Read the model definition and answer for the solid it produces. Units are mm, in the model's axes. A direction names the side the tool comes from. Coordinates: 2 decimals unless noted, no trailing zeros. Write each loop counter-clockwise with the first axis right and the second up, starting at its lowest first coordinate (ties: lowest second). Pieces come first, ordered by that corner, then holes. Notation, with made-up numbers: (-13.5, 42.25) -> (4.5, 42.25) arc R21 cw to (4.5, 77.25) -> close; hole circle Ø1 at (33.25, 58.5). An arc over 180 degrees is marked (long way). Return JSON: item names as keys, results as strings.
from build123d import *

# Parameters (mm, degrees)
ESQUISSE1_R             = 4
BOSS_EXTRU_1_DEPTH      = 3
ESQUISSE2_W             = 4.5
ESQUISSE2_H             = 4.5
BOSS_EXTRU_2_DEPTH      = 9
ESQUISSE3_W             = 2.4
ESQUISSE3_H             = 2.4
ENL_V_MAT_EXTRU_1_DEPTH = 3
CONG_1_R                = 1
CONG_2_R                = 0.5


with BuildPart() as part:
    # Esquisse1 → Boss.-Extru.1 (new body)
    with BuildSketch(Plane.XY):
        Circle(ESQUISSE1_R)
    extrude(amount=BOSS_EXTRU_1_DEPTH)

    # Esquisse2 → Boss.-Extru.2 (add)
    with BuildSketch(Plane.XY.offset(3)):
        Rectangle(ESQUISSE2_W, ESQUISSE2_H)
    extrude(amount=BOSS_EXTRU_2_DEPTH)

    # Esquisse3 → Enlèv. mat.-Extru.1 (cut)
    with BuildSketch(Plane.XY.offset(12)):
        Rectangle(ESQUISSE3_W, ESQUISSE3_H)
    extrude(amount=-ENL_V_MAT_EXTRU_1_DEPTH, mode=Mode.SUBTRACT)

    # Congé1
    cong_1_edges = [part.edges().sort_by_distance(p)[0] for p in [
        (-2.25, 2.25, 7.5),
        (-2.25, -2.25, 7.5),
        (2.25, -2.25, 7.5),
        (2.25, 2.25, 7.5),
    ]]
    fillet(cong_1_edges, radius=CONG_1_R)

    # Congé2
    cong_2_edges = [part.edges().sort_by_distance(p)[0] for p in [
        (-4, 0, 0),
    ]]
    fillet(cong_2_edges, radius=CONG_2_R)


solid = part.part
1. Flat-ended cylindrical pins translate along their axes: pin 1 Ø4 at (x, z) = (2, 4.5) entering from -Y; pin 2 Ø0.8 at (x, z) = (0.5, 6) entering from -Y; pin 3 Ø3 at (x, z) = (-0.5, 5.5) entering from +Y. Find the tip coordinate at first contact, or state that the pin passes through.
Taken from the geometry:
{"pin 1": "stops at y = -3.94", "pin 2": "stops at y = -2.25", "pin 3": "stops at y = 2.25"}
2. Consider L1, parallel to Y at x = -0.25, z = 5.75; L2, parallel to Z at x = -1.5, y = -2.25. Determine where each line is inside the solid, lowest interval first.
Taken from the geometry:
{"L1": "y = -2.25 to 2.25", "L2": "z = 0 to 3"}
3. A tool of negligible diameter and unlimited length cuts with its end or side. For faces 1 (the face through (-1.949, 1.965, 7.563)), 2 (the face through (0, -2.25, 7)), 3 (the face through (0, 2.25, 7)), 4 (the face through (2.25, 0, 7)), 5 (the face through (0, -1.2, 11)), from which of +Z, -Z, +X, -X, +Y, -Y can it reach the whole face along a straight path? Write none if from no direction.
Taken from the geometry:
{"face 1": "+Z, -X, +Y", "face 2": "+Z, +X, -X, -Y", "face 3": "+Z, +X, -X, +Y", "face 4": "+Z, +X, +Y, -Y", "face 5": "+Z"}
4. For a pull along X with two mould halves and no side action, classify faces 6 (the face through (1.949, -1.965, 7.563)), 7 (the face through (-1.949, -1.965, 7.563)), 8 (the face through (1.2, 0, 11)), 9 (the face through (3, 0, 3)) as +X half, -X half, draft (parallel to the pull), parting line (faces both ways), or undercut.
Taken from the geometry:
{"face 6": "+X half", "face 7": "-X half", "face 8": "undercut", "face 9": "draft"}
5. The part is cut by section D-D (z = 8.5). Determine the outline of the cut face in (x, y), then the cut area to 3 significant figures.
Taken from the geometry:
{"outline": "(-2.25, -1.25) arc R1 ccw to (-1.25, -2.25) -> (1.25, -2.25) arc R1 ccw to (2.25, -1.25) -> (2.25, 1.25) arc R1 ccw to (1.25, 2.25) -> (-1.25, 2.25) arc R1 ccw to (-2.25, 1.25) -> close", "area": "19.4 mm2"}
6. The part is cut by section A-A (z = 11.25). Determine the outline of the cut face in (x, y).
Taken from the geometry:
{"outline": "(-2.25, -1.25) arc R1 ccw to (-1.25, -2.25) -> (1.25, -2.25) arc R1 ccw to (2.25, -1.25) -> (2.25, 1.25) arc R1 ccw to (1.25, 2.25) -> (-1.25, 2.25) arc R1 ccw to (-2.25, 1.25) -> close; hole (-1.2, -1.2) -> (1.2, -1.2) -> (1.2, 1.2) -> (-1.2, 1.2) -> close"}
7. The part is cut by section B-B (x = 0). Determine the outline of the cut face in (y, z).
Taken from the geometry:
{"outline": "(-4, 0.5) arc R0.5 ccw to (-3.5, 0) -> (3.5, 0) arc R0.5 ccw to (4, 0.5) -> (4, 3) -> (2.25, 3) -> (2.25, 12) -> (1.2, 12) -> (1.2, 9) -> (-1.2, 9) -> (-1.2, 12) -> (-2.25, 12) -> (-2.25, 3) -> (-4, 3) -> close"}
